Part model, mm, in its own coordinate system. Face numbers are marked on the shaded views. A direction names the side the tool comes from. Round coordinates to 2 decimals unless told otherwise and drop trailing zeros. Order: outer loops, then holes, each group sorted by start corner. A loop starts at its lowest first (then second) coordinate and runs counter-clockwise, first axis right, second up. Notation, with made-up numbers: M 68,11.25 L 119,11.25 A11 ccw 119,16.25 Z; hole C 62,46 d2. An arc over 180 degrees is marked long. One line per question, with ' | ' between items.
from build123d import *

# Parameters (mm, degrees)
EXTRUDE_472_DEPTH        = 9
CUT_EXTRUDE_914_DEPTH    = 46.672748987
EXTRUDE_3_DEPTH          = 18
CUT_EXTRUDE_3_DEPTH      = 46.564039844
EXTRUDE_5_DEPTH          = 9
SWEEP_START              = -4.881222858
SWEEP_1_DEPTH            = 13.189100313
SKETCH_5_R               = 3.5
EXTRUDE_2_DEPTH          = 6
SKETCH_11_W              = 23.723512942
SKETCH_11_H              = 14
CUT_EXTRUDE_4_DEPTH      = 3
SKETCH_12_W              = 6
SKETCH_12_H              = 2.5
EXTRUDE_4_DEPTH          = 10
HOLE_WIZARD_M2_5_2_D     = 2.05
HOLE_WIZARD_M2_5_2_DEPTH = 2.5
HOLE_WIZARD_M2_5_2_TIP   = 0.615882135


with BuildPart() as part:
    # 草图1 → Extrude 472 (new, symmetric)
    with BuildSketch(Plane.XY):
        with BuildLine():
            Line((0, 9), (32, 9))
            ThreePointArc((32, 9), (41, 0), (32, -9))
            Line((32, -9), (0, -9))
            Line((0, -9), (0, 9))
        make_face()
    extrude(amount=EXTRUDE_472_DEPTH, both=True)

    # 草图13 → Cut-Extrude 914 (cut, through all)
    with BuildSketch(Plane.XY.offset(9)):
        with BuildLine():
            Line((5, -9), (32, -9))
            ThreePointArc((32, -9), (39.193747285, -5.408326913), (40.645808233, 2.5))
            Line((40.645808233, 2.5), (32.896719487, 0))
            Line((32.896719487, 0), (10.196152423, 0))
            Line((10.196152423, 0), (5, -9))
        make_face()
    extrude(amount=-CUT_EXTRUDE_914_DEPTH, mode=Mode.SUBTRACT)

    # 草图6 → 凸台-拉伸3 (add)
    with BuildSketch(Plane.XY.offset(9)):
        with BuildLine():
            Line((28, 10), (8.5, 10))
            ThreePointArc((8.5, 10), (7.153708798, 9.740728004), (6, 9))
            Line((6, 9), (30.5, 9))
            ThreePointArc((30.5, 9), (29.346291202, 9.740728004), (28, 10))
        make_face()
    extrude(amount=-EXTRUDE_3_DEPTH)

    # 草图7 → 切除-拉伸3 (cut, through all)
    with BuildSketch(Plane.XY.offset(9)):
        Polygon((2.121320344, 9), (0, 9), (0, 6.878679656), align=None)
    extrude(amount=-CUT_EXTRUDE_3_DEPTH, mode=Mode.SUBTRACT)

    # 草图14 → 凸台-拉伸5 (add, symmetric)
    with BuildSketch(Plane.XY):
        Polygon((11.775875797, 0), (8.711698025, -2.571150439), (8.711698025, 0), align=None)
    extrude(amount=EXTRUDE_5_DEPTH, both=True)

    # 切除-扫描1: read off the stored shape, not the designer's step
    # 切除-扫描1 outline → 切除-扫描1 (cut)
    with BuildSketch(Plane(origin=(0, 0, 0), x_dir=(0.7087101663277271, 0.7054997520507894, 0), z_dir=(0.7054997520507895, -0.708710166327727, 0)).offset(SWEEP_START)):
        with BuildLine():
            add(Edge.make_bspline(
                [(7.598390407, 0), (7.598390407, 2.5), (5.107415447, 2.5), (5.107415447, 0), (5.107415447, -2.5), (7.598390407, -2.5), (7.598390407, 0)],
                knots=[0, 0, 0, 0, 0.5, 0.5, 0.5, 1, 1, 1, 1], degree=3, weights=[1, 0.333333333, 0.333333333, 1, 0.333333333, 0.333333333, 1]))
        make_face()
    extrude(amount=SWEEP_1_DEPTH, mode=Mode.SUBTRACT)

    # 草图5 → 凸台-拉伸2 (add, symmetric)
    with BuildSketch(Plane.XY):
        with BuildLine():
            Line((0, 7), (-12, 7))
            ThreePointArc((-12, 7), (-19, 0), (-12, -7))
            Line((-12, -7), (0, -7))
            Line((0, -7), (0, 7))
        make_face()
        with Locations((-12, 0)):
            Circle(SKETCH_5_R, mode=Mode.SUBTRACT)
    extrude(amount=EXTRUDE_2_DEPTH, both=True)

    # 草图11 → 切除-拉伸4 (cut, symmetric)
    with BuildSketch(Plane.XY):
        with Locations((-11.861756471, 0)):
            Rectangle(SKETCH_11_W, SKETCH_11_H)
    extrude(amount=CUT_EXTRUDE_4_DEPTH, both=True, mode=Mode.SUBTRACT)

    # 草图12 → 凸台-拉伸4 (add)
    with BuildSketch(Plane.ZY):
        with Locations((0, -5.75)):
            Rectangle(SKETCH_12_W, SKETCH_12_H)
    extrude(amount=EXTRUDE_4_DEPTH)

    # M2.5 螺纹孔2
    with Locations(Plane(origin=(19.775875797, 0, 0), x_dir=(0, 0, -1), z_dir=(0, -1, 0))):
        with Locations((0, 0)):
            Hole(HOLE_WIZARD_M2_5_2_D / 2, depth=HOLE_WIZARD_M2_5_2_DEPTH)
            with Locations((0, 0, -(HOLE_WIZARD_M2_5_2_DEPTH + HOLE_WIZARD_M2_5_2_TIP / 2))):  # 118° drill point
                Cone(0, HOLE_WIZARD_M2_5_2_D / 2, HOLE_WIZARD_M2_5_2_TIP, mode=Mode.SUBTRACT)


solid = part.part
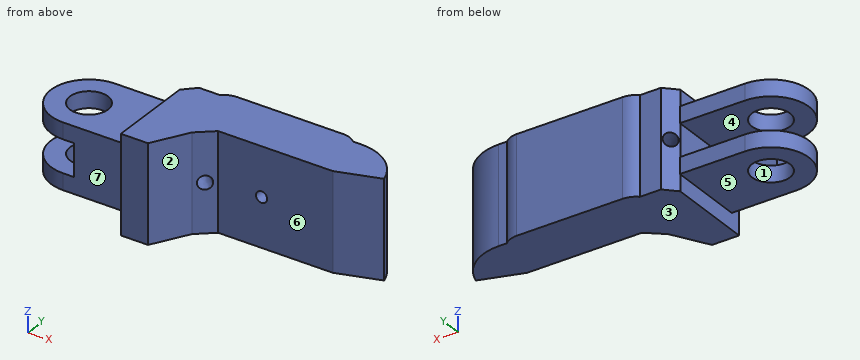
1) Drop flat-ended pins along their axis: pin 1 (4 mm diameter, centred on x = -7.5, y = 0.5, fed in from +Z); pin 2 (8 mm diameter, centred on x = -12, y = 0, fed in from -Z); pin 3 (2.5 mm diameter, centred on x = -3, z = 4.5, fed in from +Y). Give the stop position or say it passes through.
The answers:
pin 1: stops at z = 6 | pin 2: stops at z = -6 | pin 3: stops at y = 7
2) Saw through at D-D (z = 7.25). List the corners of the cut face in (x, y) (3 decimals), plus the area to 3 significant figures.
The answers:
outline: M 0,-9 L 5,-9 L 8.712,-2.571 L 11.776,0 L 32.897,0 L 40.646,2.5 A9 ccw 32,9 L 30.5,9 A3.625 ccw 28,10 L 8.5,10 A3.625 ccw 6,9 L 2.121,9 L 0,6.879 Z | area: 432 mm²
3) Which spindle directions (+Z, -Z, +X, -X, +Y, -Y) get a long thin tool onto all of the face, cutting with end or side? Do the marked faces 4, 5, 6 and 7. Say none if no direction does.
The answers:
face 4: -X, +Y | face 5: -Z, -X, +Y, -Y | face 6: +Z, -Z, +X, -Y | face 7: +Z, -Z, -X, -Y
4) Saw through at B-B (y = 1). Give the number of separate pieces and of enclosed holes in the cut face, plus the area to 3 significant figures.
The answers:
separate pieces: 3 | enclosed holes: 2 | area: 711 mm²
5) Two-plate mould, pull along X, no slides. Class the marked faces 1, 2 and 3: released by +X, released by -X, zero draft, split by the parting line, or undercut.
The answers:
face 1: undercut | face 2: released by +X | face 3: zero draft
6) Probe line 1 (Z direction, x = -6.5, y = -3.5); line 2 (Y direction, x = -3, z = 0); line 3 (Y direction, x = 4.5, z = -8). List the from-to ranges inside material, lowest first. Write a range as [from, to].
The answers:
line 1: z = [-6, -3], [3, 6] | line 2: y = [-7, -4.5] | line 3: y = [-9, 9]
7) Saw through at C-C (y = -5.25). List the corners of the cut face in (x, z), plus the area to 3 significant figures.
The answers:
outline: M -16.63,-6 L 0,-6 L 0,-9 L 7.17,-9 L 7.17,9 L 0,9 L 0,6 L -16.63,6 L -16.63,3 L -10,3 L -10,-3 L -16.63,-3 Z | area: 289 mm²
8) Saw through at A-A (z = -2). List the corners of the cut face in (x, y) (3 decimals).
The answers:
outline: M -10,-7 L 0,-7 L 0,-9 L 5,-9 L 8.712,-2.571 L 11.776,0 L 32.897,0 L 40.646,2.5 A9 ccw 32,9 L 30.5,9 A3.625 ccw 28,10 L 8.5,10 A3.625 ccw 6,9 L 2.121,9 L 0,6.879 L 0,-4.5 L -10,-4.5 Z
